from build123d import *

# Parameters (mm, degrees)
BOSS_EXTRUDE1_DEPTH      = 70.958248
BOSS_EXTRUDE1_DEPTH_BACK = 9.041752
SKETCH3_R                = 5.515432893
CUT_EXTRUDE1_DEPTH       = 22
SKETCH4_W                = 56.790594551
SKETCH4_H                = 75.94381824
CUT_EXTRUDE2_DEPTH       = 31
SKETCH5_W                = 75
SKETCH5_H                = 75.94381824
CUT_EXTRUDE3_DEPTH       = 51


with BuildPart() as part:
    # Sketch1 → Boss-Extrude1 (new, two sides: drawn at the far end of the back side and taken through both)
    with BuildSketch(Plane.XY.offset(-BOSS_EXTRUDE1_DEPTH_BACK)):
        Polygon((97.04953752, 44.971194673), (97.04953752, 47.971194673), (88.459572821, 47.971194673), (88.459572821, 100.803034254), (0, 100.803034254), (0, 78.655691188), (-46.687150509, 78.655691188), (-46.687150509, 44.971194673), align=None)
    extrude(amount=BOSS_EXTRUDE1_DEPTH + BOSS_EXTRUDE1_DEPTH_BACK)

    # Sketch3 → Cut-Extrude1 (cut)
    with BuildSketch(Plane.ZY.offset(46.687150509)):
        with Locations(Location((32.421386427, 59.322946804, 0), (0, 0, 270))):
            Circle(SKETCH3_R)
    extrude(amount=-CUT_EXTRUDE1_DEPTH, mode=Mode.SUBTRACT)

    # Sketch4 → Cut-Extrude2 (cut)
    with BuildSketch(Plane(origin=(0, 44.971194673, 0), x_dir=(-1, 0, 0), z_dir=(0, -1, 0))):
        with Locations((16.345759756, -30.684219126)):
            Rectangle(SKETCH4_W, SKETCH4_H)
    extrude(amount=-CUT_EXTRUDE2_DEPTH, mode=Mode.SUBTRACT)

    # Sketch5 → Cut-Extrude3 (cut)
    with BuildSketch(Plane(origin=(0, 44.971194673, 0), x_dir=(-1, 0, 0), z_dir=(0, -1, 0))):
        with Locations((-49.54953752, -30.684219126)):
            Rectangle(SKETCH5_W, SKETCH5_H)
    extrude(amount=-CUT_EXTRUDE3_DEPTH, mode=Mode.SUBTRACT)


solid = part.part
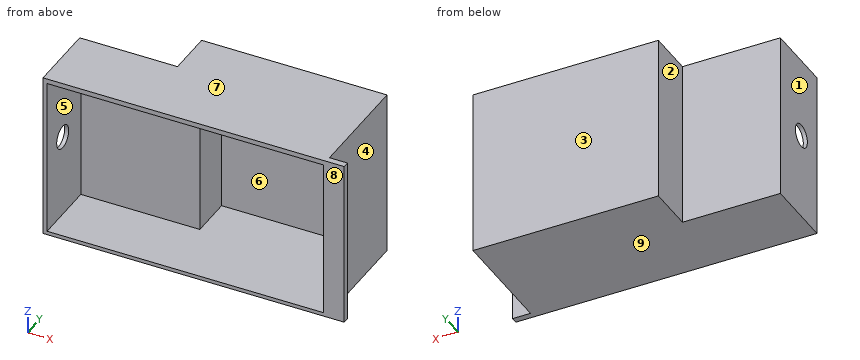
Source: CAD feature listing. Evaluate the final solid. Frame: model axes, mm. Face numbers are marked on the shaded views. A direction names the side the tool comes from. Round coordinates to 2 decimals unless told otherwise and drop trailing zeros. Order: outer loops, then holes, each group sorted by start corner. A loop starts at its lowest first (then second) coordinate and runs counter-clockwise, first axis right, second up. Notation, with made-up numbers: (-31.75, 3.5) - (6.25, 3.5) arc R22 ccw to (6.25, 18.5) - close; hole circle Ø6 at (-39, 4). An arc over 180 degrees is marked (long way). Use a Markdown table: item, result. Add a question column.
1. Line query: probe 1 along Z at (x, y) = (-9.5, 63.5); probe 2 along X at (y, z) = (89, 20); probe 3 along X at (y, z) = (64, 48). Output: solid intervals per line, ascending.
2. Section query A-A (y = 93). Return the cut outline in (x, z).
3. Section query C-C (x = 40). Return the cut outline in (y, z).
4. Mould query, pull axis Z, two halves, no side actions, for the marked faces 6, 7, 8 and 9. Classes: +Z half, -Z half, draft (parallel to the pull), parting line (faces both ways), or undercut.
5. Set-up query: the marked faces 1, 2, 3, 4 and 5. Return all of +Z, -Z, +X, -X, +Y, -Y with unobstructed straight access to the full face (end or side cutting, diameter ignored); none if empty.
6. Section query B-B (z = 2). Return the cut outline in (x, y), then the cut area to 3 significant figures.
7. First-contact query: pin 1 (10 mm diameter, centred on y = 53.5, z = 42, fed in from +X); pin 2 (1.5 mm diameter, centred on x = -19, y = 80, fed in from +Z); pin 3 (1.5 mm diameter, centred on x = -24.5, z = 3.5, fed in from +Y); pin 4 (2.5 mm diameter, centred on x = 95, z = 12.5, fed in from +Y). Flat tips, straight axial feed; report the tip coordinate or a pass-through.
8. Section query D-D (z = 36). Return the cut outline in (x, y).
Derived:
| question | item | result |
|---|---|---|
| 1 | probe 1 | -9.04 to -7.29, 68.66 to 70.96 |
| 1 | probe 2 | 0 to 12.05, 87.05 to 88.46 |
| 1 | probe 3 | -46.69 to -44.74, 87.05 to 88.46 |
| 2 | outline | (0, -9.04) - (88.46, -9.04) - (88.46, 70.96) - (0, 70.96) - close; hole (12.05, -7.29) - (87.05, -7.29) - (87.05, 68.66) - (12.05, 68.66) - close |
| 3 | outline | (44.97, -9.04) - (100.8, -9.04) - (100.8, 70.96) - (44.97, 70.96) - (44.97, 68.66) - (95.97, 68.66) - (95.97, -7.29) - (44.97, -7.29) - close |
| 4 | face 6 | undercut |
| 4 | face 7 | +Z half |
| 4 | face 8 | draft |
| 4 | face 9 | -Z half |
| 5 | face 1 | +Z, -Z, -X, +Y, -Y |
| 5 | face 2 | +Z, -Z, -X, +Y |
| 5 | face 3 | +Z, -Z, +X, -X, +Y |
| 5 | face 4 | +Z, -Z, +X, +Y |
| 5 | face 5 | -Y |
| 6 | outline | (-46.69, 44.97) - (-44.74, 44.97) - (-44.74, 75.97) - (12.05, 75.97) - (12.05, 95.97) - (87.05, 95.97) - (87.05, 44.97) - (97.05, 44.97) - (97.05, 47.97) - (88.46, 47.97) - (88.46, 100.8) - (0, 100.8) - (0, 78.66) - (-46.69, 78.66) - close |
| 6 | area | 952 mm2 |
| 7 | pin 1 | x = 88.46 |
| 7 | pin 2 | through |
| 7 | pin 3 | y = 78.66 |
| 7 | pin 4 | y = 47.97 |
| 8 | outline | (-46.69, 44.97) - (-44.74, 44.97) - (-44.74, 55.13) - (-46.69, 55.13) - close; (-46.69, 63.52) - (-44.74, 63.52) - (-44.74, 75.97) - (12.05, 75.97) - (12.05, 95.97) - (87.05, 95.97) - (87.05, 44.97) - (97.05, 44.97) - (97.05, 47.97) - (88.46, 47.97) - (88.46, 100.8) - (0, 100.8) - (0, 78.66) - (-46.69, 78.66) - close |
